The listing builds one solid part. Answer for the finished solid, in the listing's coordinates (mm). Face numbers are marked on the shaded views. A direction names the side the tool comes from. Round coordinates to 2 decimals unless told otherwise and drop trailing zeros. Loops run counter-clockwise (first coordinate to the right, second up) from the corner with the lowest first, then second, coordinate; pieces in that order, holes last. Notation, with made-up numbers: (11, -37.5) -> (68, -37.5) arc R8 ccw to (68, -30.5) -> close; hole circle Ø7 at (53, -5). An arc over 180 degrees is marked (long way). One line per question, with ' | ' between items.
from build123d import *

# Parameters (mm, degrees)
F0_W     = 76.2
F0_H     = 76.2
F1_DEPTH = 76.2
F2_T     = -2.54
F4_D     = 6.35
F6_D     = 6.35


with BuildPart() as f1:
    # F0 (on Front) → F1 (new body)
    with BuildSketch(Plane.XZ):
        with Locations((38.1, -38.1)):
            Rectangle(F0_W, F0_H)
    extrude(amount=F1_DEPTH)

    # F2
    f2_openings = [f1.faces().sort_by_distance(p)[0] for p in [
        (38.1, -76.2, -38.1),
    ]]
    offset(amount=F2_T, openings=f2_openings)

    # F4 (through all)
    with Locations(Plane(origin=(0, 0, 0), x_dir=(-1, 0, 0), z_dir=(0, 1, 0))):
        with Locations((-69.99965, -35.934076)):
            Hole(F4_D / 2)

    # F6 (through all)
    with Locations(Plane.XZ.offset(2.54)):
        with Locations((5.889626, -35.706378)):
            Hole(F6_D / 2)


solid = f1.part
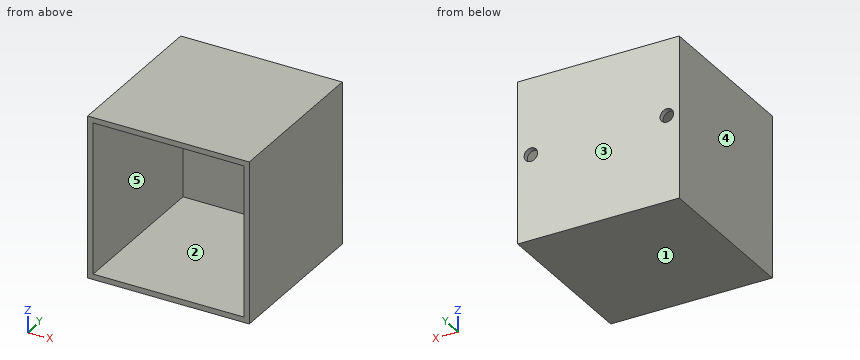
Q1. A cutting plane is placed at C-C on y = -37.5. Give the vertices of the cut face in (x, z), plus the area to 3 significant figures.
Numbers:
outline: (0, -76.2) -> (76.2, -76.2) -> (76.2, 0) -> (0, 0) -> close; hole (2.54, -73.66) -> (73.66, -73.66) -> (73.66, -2.54) -> (2.54, -2.54) -> close | area: 748 mm^2
Q2. For the marked faces 1 and 2, determine the directions among +Z, -Z, +X, -X, +Y, -Y from which every point of the face is accessible in a straight line to the end or side of a thin tool.
Numbers:
face 1: -Z, +X, -X, +Y, -Y | face 2: -Y
Q3. A cutting plane is placed at D-D on x = 71. Give the vertices of the cut face in (y, z), plus the area to 3 significant figures.
Numbers:
outline: (-76.2, -76.2) -> (0, -76.2) -> (0, -38.95) -> (-2.54, -38.95) -> (-2.54, -73.66) -> (-76.2, -73.66) -> close; (-76.2, -2.54) -> (-2.54, -2.54) -> (-2.54, -32.92) -> (0, -32.92) -> (0, 0) -> (-76.2, 0) -> close | area: 552 mm^2
Q4. A cutting plane is placed at B-B on x = 55.5. Give the vertices of the cut face in (y, z), plus the area to 3 significant figures.
Numbers:
outline: (-76.2, -76.2) -> (0, -76.2) -> (0, 0) -> (-76.2, 0) -> (-76.2, -2.54) -> (-2.54, -2.54) -> (-2.54, -73.66) -> (-76.2, -73.66) -> close | area: 568 mm^2
Q5. Given pin 1 Ø21.5 at (x, z) = (39, -40.5) entering from -Y; pin 2 Ø4 at (x, z) = (70, -35.93) entering from +Y, each flat-ended and moving along its own axis, determine where each tip first touches the part or whether it passes through.
Numbers:
pin 1: y = -2.54 | pin 2: through
Q6. Find the intervals of material crossed by line 1 (X direction, y = -47, z = -51.5); line 2 (Z direction, x = 29.5, y = -39); line 3 (Y direction, x = 61, z = -35.5), in increasing order. Write a range as from..to.
Numbers:
line 1: 0..2.54, 73.66..76.2 | line 2: -76.2..-73.66, -2.54..0 | line 3: -2.54..0
Q7. For a pull along X with two mould halves and no side action, classify the marked faces 3, 4 and 5 as pulls with the +X half, pulls with the -X half, needs draft (parallel to the pull), parting line crosses it, or undercut.
Numbers:
face 3: needs draft | face 4: pulls with the -X half | face 5: undercut
Q8. A cutting plane is placed at A-A on z = -27. Give the vertices of the cut face in (x, y), plus the area to 3 significant figures.
Numbers:
outline: (0, -76.2) -> (2.54, -76.2) -> (2.54, -2.54) -> (73.66, -2.54) -> (73.66, -76.2) -> (76.2, -76.2) -> (76.2, 0) -> (0, 0) -> close | area: 568 mm^2
